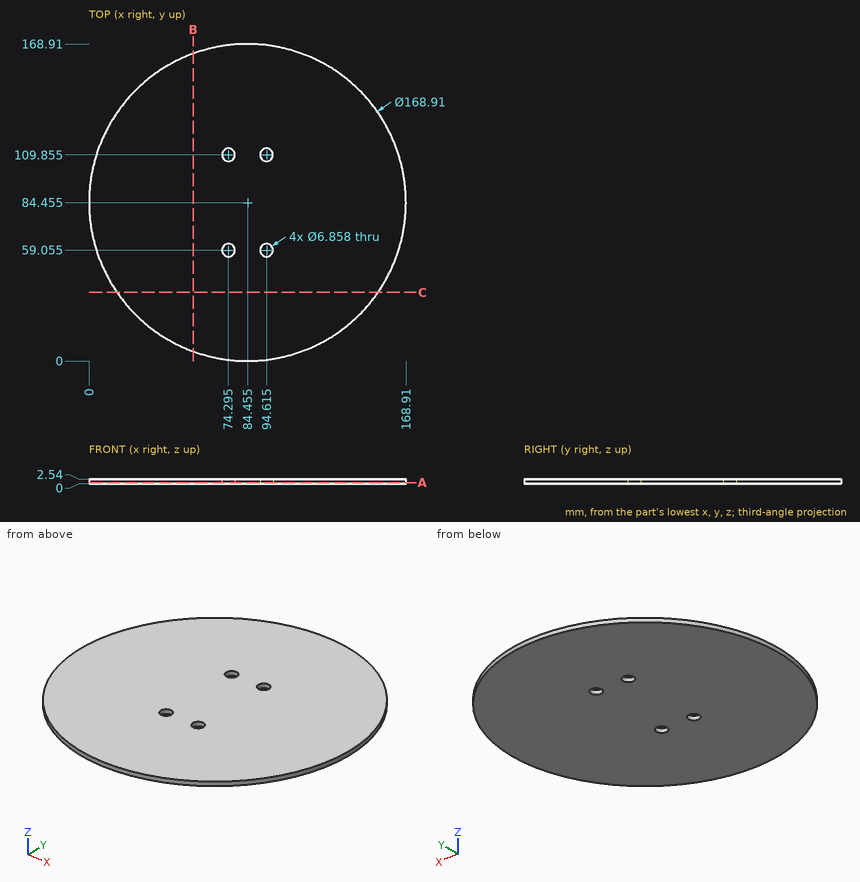
Job drawing, mm, ordinate dimensions from the low corner. One solid piece. Give positions to 0.01 mm unless a question says otherwise; leave off trailing zeros. Loops run counter-clockwise (first coordinate to the right, second up) from the corner with the lowest first, then second, coordinate; pieces in that order, holes last. Notation, with made-up numbers: (18.5, 47.25) -> (32.5, 47.25) arc R10 cw to (32.5, 58.25) -> close; hole circle Ø4 at (29.5, -38). An arc over 180 degrees is marked (long way). Use a Markdown table: item, result. Add a question column.
(1) Slice it at B-B on x = 55.5. List the corners of the cut face in (y, z).
(2) Slice it at A-A on z = 0.65. List the corners of the cut face in (x, y) (3 decimals), and give its area (3 significant figures).
(3) Wall check: line 1 along X through (y, z) = (112, 2.4); line 2 along Y through (x, z) = (132, 1.35); line 3 along X through (y, z) = (131.5, 1.05). Give the ranges that are in metal, low to high.
(4) Drop a flat-ended pin along its axis: pin 1 Ø9 at (x, y) = (94.615, 59.055) entering from +Z. Give the stop position or say it passes through.
(5) Slice it at C-C on y = 36.5. List the corners of the cut face in (x, z), and give its area (3 significant figures).
Filled sheet:
| question | item | result |
|---|---|---|
| 1 | outline | (5.12, 0) -> (163.79, 0) -> (163.79, 2.54) -> (5.12, 2.54) -> close |
| 2 | outline | circle Ø168.91 at (84.455, 84.455); hole circle Ø6.858 at (74.295, 59.055); hole circle Ø6.858 at (74.295, 109.855); hole circle Ø6.858 at (94.615, 59.055); hole circle Ø6.858 at (94.615, 109.855) |
| 2 | area | 22,300 mm2 |
| 3 | line 1 | 4.62 to 71.62, 76.97 to 91.94, 97.29 to 164.29 |
| 3 | line 2 | 14.65 to 154.26 |
| 3 | line 3 | 14.32 to 154.59 |
| 4 | pin 1 | z = 2.54 |
| 5 | outline | (14.94, 0) -> (153.97, 0) -> (153.97, 2.54) -> (14.94, 2.54) -> close |
| 5 | area | 353 mm2 |
